Geometry check sheet. Reference: the model listing, model coordinates, mm. A direction names the side the tool comes from. Round coordinates to 2 decimals unless told otherwise and drop trailing zeros. Write each loop counter-clockwise with the first axis right and the second up, starting at its lowest first coordinate (ties: lowest second). Pieces come first, ordered by that corner, then holes. Notation, with made-up numbers: M 25.5,-25 L 65.5,-25 A25 ccw 65.5,1 Z; hole C 65.25,51.25 d11. An arc over 180 degrees is marked long. Put each result on its own line as item: value. Start each with the question number.
(1) Section check B-B on x = 114. Record the cut outline in (y, z), then the cut area to 3 significant figures.
(2) Mould release check, pull along X, two halves, no side actions. Record for faces 1 (the flat face through (99, 2, -65)), 2 (the flat face through (-2, -21, 0)), 3 (the flat face through (99, 0, -53)): pulls with the +X half, pulls with the -X half, needs draft (parallel to the pull), parting line crosses it, or undercut.
(3) Material ranges on probe 1 along Y at (x, z) = (-1, 0); probe 2 along Y at (x, z) = (91.5, -86); probe 3 along Y at (x, z) = (138, -1), recorded low to high.
(4) Tool access check on faces 4 (the flat face through (0, -23, 0)), 5 (the cylindrical face through (-1, -43, 0)). Record the directions out of +Z, -Z, +X, -X, +Y, -Y that give a thin tool (end or side, any length) a straight path to the whole face; none if there is none.
(5) Section check A-A on y = -4. Record the cut outline in (x, z), then the cut area to 3 significant figures.
(6) Section check D-D on z = -55. Record the cut outline in (x, y).
(7) Section check C-C on z = -123. Record the cut outline in (x, y).
(8) Gauge pin test, flat ends, axial feed: pin 1 (3 mm diameter, centred on x = 58, z = -52.5, fed in from +Y); pin 2 (5 mm diameter, centred on y = -41, z = 0, fed in from -X). Record the tip position at first contact, or that the pin passes through.
from build123d import *

# Parameters (mm, degrees)
SKETCH2_R           = 2
BOSS_EXTRUDE1_DEPTH = 2
SKETCH4_W           = 200
SKETCH4_H           = 20
BOSS_EXTRUDE4_DEPTH = 2
SKETCH7_W           = 2
SKETCH7_H           = 20
BOSS_EXTRUDE5_DEPTH = 50
FILLET1_R           = 5
SKETCH9_R           = 2
CUT_EXTRUDE1_DEPTH  = 250


with BuildPart() as part:
    # Sketch2 → Boss-Extrude1 (new body)
    with BuildSketch(Plane(origin=(0, 0, 0), x_dir=(1, 0, 0), z_dir=(0, 1, 0))):
        Polygon((200, 0), (200, 10), (100, 150), (0, 10), (0, 0), (0, -10), (200, -10), align=None)
        with Locations(Location((100, 137.477270849, 0), (0, 0, 270))):
            Circle(SKETCH2_R, mode=Mode.SUBTRACT)
    extrude(amount=BOSS_EXTRUDE1_DEPTH)

    # Sketch4 → Boss-Extrude4 (add)
    with BuildSketch(Plane(origin=(0, 2, 0), x_dir=(1, 0, 0), z_dir=(0, 1, 0))):
        with Locations((100, 0)):
            Rectangle(SKETCH4_W, SKETCH4_H)
    extrude(amount=BOSS_EXTRUDE4_DEPTH)

    # Sketch7 → Boss-Extrude5 (add)
    with BuildSketch(Plane(origin=(0, 4, 0), x_dir=(1, 0, 0), z_dir=(0, 1, 0))):
        with Locations((-1, 0)):
            Rectangle(SKETCH7_W, SKETCH7_H)
        with Locations((201, 0)):
            Rectangle(SKETCH7_W, SKETCH7_H)
    extrude(amount=-BOSS_EXTRUDE5_DEPTH)

    # Fillet1
    fillet1_edges = [part.edges().sort_by_distance(p)[0] for p in [
        (-1, -46, 10),
        (-1, -46, -10),
        (201, -46, -10),
        (201, -46, 10),
    ]]
    fillet(fillet1_edges, radius=FILLET1_R)

    # Sketch9 → Cut-Extrude1 (cut)
    with BuildSketch(Plane.ZY.offset(2)):
        with Locations((0, -41)):
            Circle(SKETCH9_R)
    extrude(amount=-CUT_EXTRUDE1_DEPTH, mode=Mode.SUBTRACT)


solid = part.part
Answers follow:
1. outline: M 0,-130.4 L 2,-130.4 L 2,-10 L 4,-10 L 4,10 L 0,10 Z
1. area: 321 mm^2
2. face 1: needs draft
2. face 2: pulls with the -X half
2. face 3: undercut
3. probe 1: y = -46 to -43, -39 to 4
3. probe 2: y = 0 to 2
3. probe 3: y = 0 to 4
4. face 4: +Z, -Z, -Y
4. face 5: +X, -X
5. outline: M -2,-10 L 0,-10 L 0,10 L -2,10 Z; M 200,-10 L 202,-10 L 202,10 L 200,10 Z
5. area: 80.0 mm^2
6. outline: M 32.14,0 L 167.86,0 L 167.86,2 L 32.14,2 Z
7. outline: M 80.71,0 L 119.29,0 L 119.29,2 L 80.71,2 Z
8. pin 1: stops at y = 2
8. pin 2: stops at x = -2
